Check sheet for the drawn part. Datum: minimum x, y, z corner. Units: mm. Coordinates: 2 decimals unless noted, no trailing zeros. Write each loop counter-clockwise with the first axis right and the second up, starting at its lowest first coordinate (ties: lowest second). Pieces come first, ordered by that corner, then holes. Notation, with made-up numbers: M -29,26.5 L -10,26.5 A10 cw -10,38.5 Z; hole C -26,41 d8. An arc over 180 degrees is marked long. Answer as CSV lines item,"result". Start each with the question number.
Q1. Sectioned sample at C-C, the plane z = 100. Record the cut outline in (x, y).
Q2. Depth check by flat-ended pin: pin 1 Ø4.5 at (y, z) = (21.5, 30.5) entering from +X; pin 2 Ø6 at (x, y) = (145, 21.5) entering from -Z; pin 3 Ø8 at (x, y) = (94, 22) entering from +Z; pin 4 Ø8 at (y, z) = (17, 148.5) entering from -X. Enter the tip coordinate at first touch or a pass-through.
Q3. Sectioned sample at A-A, the plane y = 25. Record the cut outline in (x, z).
Q4. Sectioned sample at B-B, the plane x = 216. Record the cut outline in (y, z).
Q5. Thickness scan on line 1 along Z through (x, y) = (250.5, 16); line 2 along X through (y, z) = (7, 100); line 3 along Y through (x, z) = (146, 108). Record the ranges inside material, lowest first. Write a range as from..to.
Q6. Sectioned sample at D-D, the plane z = 135. Record the cut outline in (x, y), then the cut area to 3 significant figures.
Q7. Mould release check, pull along Z, two halves, no side actions. Record for the marked faces 1 and 2: pulls with the +Z half, pulls with the -Z half, needs draft (parallel to the pull), parting line crosses it, or undercut.
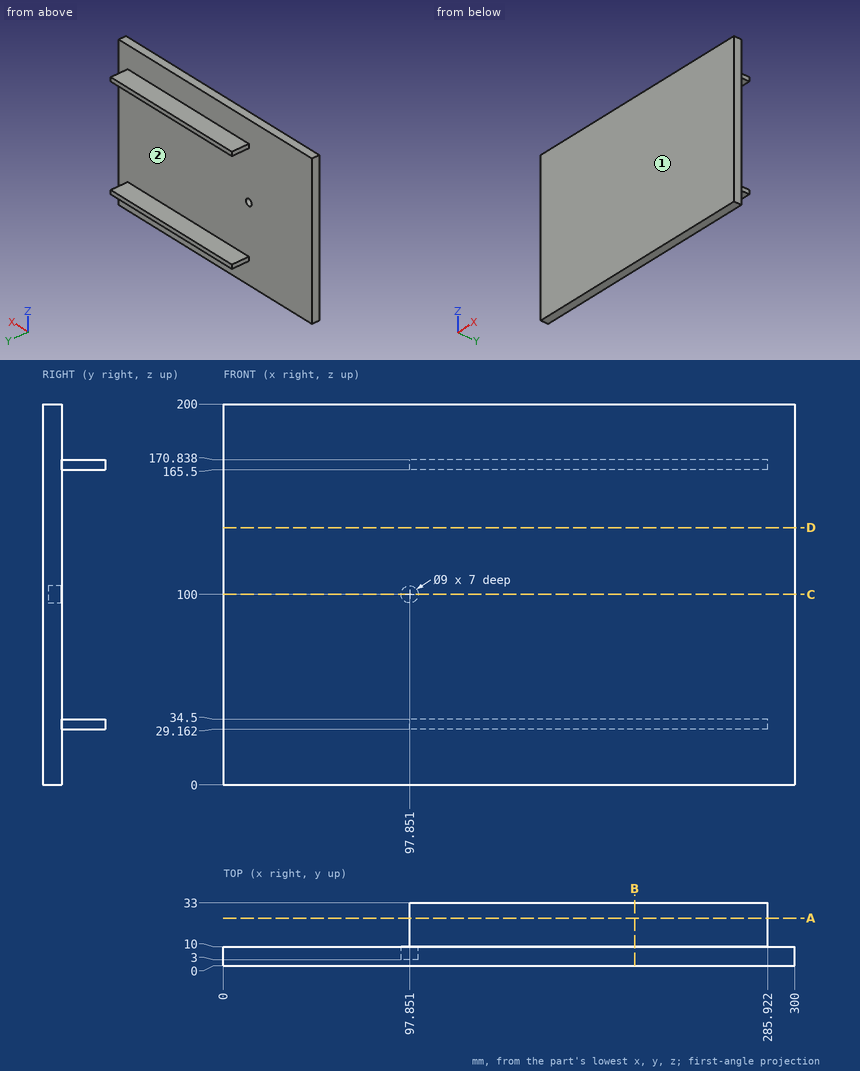
Output:
1,outline,"M 0,0 L 300,0 L 300,10 L 102.35,10 L 102.35,3 L 93.35,3 L 93.35,10 L 0,10 Z"
2,pin 1,"stops at x = 285.92"
2,pin 2,"stops at z = 29.16"
2,pin 3,"stops at z = 170.84"
2,pin 4,"passes through"
3,outline,"M 97.85,29.16 L 285.92,29.16 L 285.92,34.5 L 97.85,34.5 Z; M 97.85,165.5 L 285.92,165.5 L 285.92,170.84 L 97.85,170.84 Z"
4,outline,"M 0,0 L 10,0 L 10,29.16 L 33,29.16 L 33,34.5 L 10,34.5 L 10,165.5 L 33,165.5 L 33,170.84 L 10,170.84 L 10,200 L 0,200 Z"
5,line 1,"z = 29.16..34.5, 165.5..170.84"
5,line 2,"x = 0..93.35, 102.35..300"
5,line 3,"y = 0..10"
6,outline,"M 0,0 L 300,0 L 300,10 L 0,10 Z"
6,area,"3,000 mm^2"
7,face 1,"needs draft"
7,face 2,"undercut"
